Source: CAD feature listing. Evaluate the final solid. Frame: model axes, mm. Face numbers are marked on the shaded views. A direction names the side the tool comes from. Round coordinates to 2 decimals unless told otherwise and drop trailing zeros. Order: outer loops, then holes, each group sorted by start corner. A loop starts at its lowest first (then second) coordinate and runs counter-clockwise, first axis right, second up. Notation, with made-up numbers: M 43.5,-20 L 86.5,-20 A31 ccw 86.5,10 Z; hole C -0.5,28.5 d8. An arc over 180 degrees is marked long. Answer as CSV lines item,"result". Start each with the question number.
Item 1: Set-up query: the marked faces 3 and 4. Return all of +Z, -Z, +X, -X, +Y, -Y with unobstructed straight access to the full face (end or side cutting, diameter ignored); none if empty.
Item 2: First-contact query: P1, Ø3, axis at x = 26, y = 14.5, coming from the +Z side; P2, Ø1.5, axis at y = -8, z = 5.5, coming from the -X side; P3, Ø2, axis at x = 74.5, z = 13, coming from the +Y side. Flat tips, straight axial feed; report the tip coordinate or a pass-through.
Item 3: Pull-direction query (Y, two-part tool) for the marked faces 1 and 2; classes: +Y half, -Y half, draft (parallel to the pull), parting line (faces both ways), or undercut.
Item 4: Section query D-D on x = 16. Return the cut outline in (y, z).
Item 5: Line query: line 1 (X direction, y = -3, z = 10.25); line 2 (X direction, y = 14.5, z = 9); line 3 (X direction, y = 27, z = 2.25). Output: solid intervals per line, ascending. Write a range as [from, to].
Item 6: Section query B-B on z = 7.5. Return the cut outline in (x, y) (3 decimals).
Item 7: Section query C-C on y = -10. Return the cut outline in (x, z) (3 decimals).
Item 8: Section query A-A on y = 0. Return the cut outline in (x, z).
from build123d import *

# Parameters (mm, degrees)
F0_W      = 228.6
F0_H      = 82.804
F1_DEPTH  = 3.81
F2_R      = 36.195
F3_DEPTH  = 12.7
F4_R      = 36.195
F5_DEPTH  = 12.7
F6_R      = 31.75
F7_DEPTH  = 17.78
F8_R      = 31.75
F9_DEPTH  = 17.78
F10_W     = 6.35
F10_H     = 20.32
F11_DEPTH = 7.62
F12_W     = 6.35
F12_H     = 12.7
F13_DEPTH = 7.62
F14_W     = 6.35
F14_H     = 12.7
F15_DEPTH = 7.62


with BuildPart() as f1:
    # F0 (on Top) → F1 (new body)
    with BuildSketch(Plane.XY):
        Rectangle(F0_W, F0_H)
    extrude(amount=F1_DEPTH)

    # F2 (on face) → F3 (join)
    with BuildSketch(Plane.XY.offset(3.81)):
        with Locations((-76.315269, 0)):
            Circle(F2_R)
    extrude(amount=F3_DEPTH)

    # F4 (on face) → F5 (join)
    with BuildSketch(Plane.XY.offset(3.81)):
        with Locations((76.060459, 0)):
            Circle(F4_R)
    extrude(amount=F5_DEPTH)

    # F6 (on face) → F7 (cut)
    with BuildSketch(Plane.XY.offset(16.51)):
        with Locations((-76.315269, 0)):
            Circle(F6_R)
    extrude(amount=-F7_DEPTH, mode=Mode.SUBTRACT)

    # F8 (on face) → F9 (cut)
    with BuildSketch(Plane.XY.offset(16.51)):
        with Locations((76.060459, 0)):
            Circle(F8_R)
    extrude(amount=-F9_DEPTH, mode=Mode.SUBTRACT)

    # F10 (on face) → F11 (cut)
    with BuildSketch(Plane.XY.offset(3.81)):
        with Locations((0, -15.925558)):
            Rectangle(F10_W, F10_H)
    extrude(amount=-F11_DEPTH, mode=Mode.SUBTRACT)

    # F12 (on face) → F13 (cut)
    with BuildSketch(Plane.XY.offset(3.81)):
        with Locations((-10.712087, -19.003488)):
            Rectangle(F12_W, F12_H)
    extrude(amount=-F13_DEPTH, mode=Mode.SUBTRACT)

    # F14 (on face) → F15 (cut)
    with BuildSketch(Plane.XY.offset(3.81)):
        with Locations((10.31976, -19.003488)):
            Rectangle(F14_W, F14_H)
    extrude(amount=-F15_DEPTH, mode=Mode.SUBTRACT)


solid = f1.part
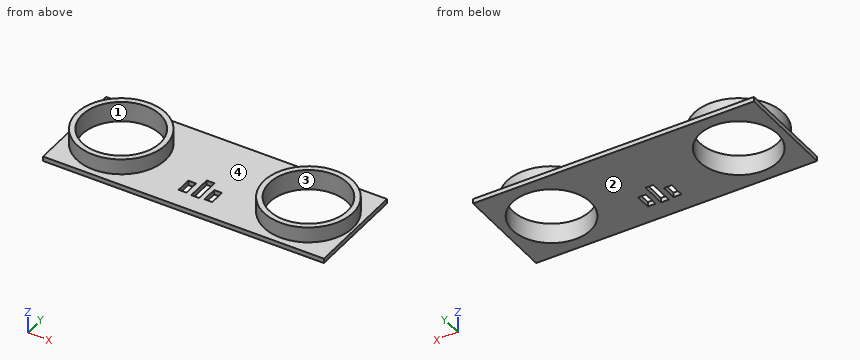
Results:
1,face 3,"+Z, -Z"
1,face 4,"+Z"
2,P1,"z = 3.81"
2,P2,"x = -111.78"
2,P3,"y = 36.19"
3,face 1,"undercut"
3,face 2,"draft"
4,outline,"M -41.4,0 L 41.4,0 L 41.4,3.81 L -41.4,3.81 Z"
5,line 1,"[-112.39, -107.92], [-44.71, -40.24], [39.99, 44.45], [107.67, 112.13]"
5,line 2,"[-109.48, -104.56], [-48.07, -43.15], [42.9, 47.81], [104.31, 109.22]"
5,line 3,"[-114.3, -93.02], [-59.61, 59.36], [92.77, 114.3]"
6,outline,"C -76.315,0 d72.39; C 76.06,0 d72.39; hole C -76.315,0 d63.5; hole C 76.06,0 d63.5"
7,outline,"M -114.3,0 L -106.449,0 L -106.449,16.51 L -111.101,16.51 L -111.101,3.81 L -114.3,3.81 Z; M -46.181,0 L -3.175,0 L -3.175,3.81 L -41.529,3.81 L -41.529,16.51 L -46.181,16.51 Z; M 3.175,0 L 45.926,0 L 45.926,16.51 L 41.274,16.51 L 41.274,3.81 L 3.175,3.81 Z; M 106.195,0 L 114.3,0 L 114.3,3.81 L 110.847,3.81 L 110.847,16.51 L 106.195,16.51 Z"
8,outline,"M -114.3,0 L -108.07,0 L -108.07,16.51 L -112.51,16.51 L -112.51,3.81 L -114.3,3.81 Z; M -44.57,0 L 44.31,0 L 44.31,16.51 L 39.87,16.51 L 39.87,3.81 L -40.12,3.81 L -40.12,16.51 L -44.57,16.51 Z; M 107.81,0 L 114.3,0 L 114.3,3.81 L 112.26,3.81 L 112.26,16.51 L 107.81,16.51 Z"
